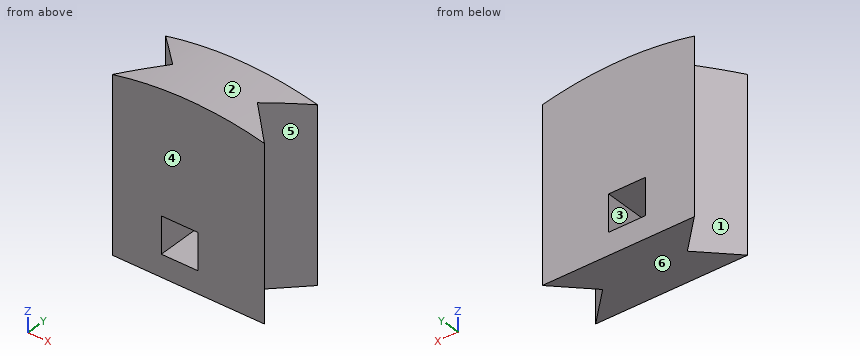
from build123d import *

# Parameters (mm, degrees)
F1_DEPTH = 47
F3_DEPTH = 25
F4_W     = 9.5
F4_H     = 9.5
F5_DEPTH = 25


with BuildPart() as f1:
    # F0 (on Top) → F1 (new body)
    with BuildSketch(Plane.XY):
        Polygon((8.75, 8.75), (0, 0), (39.5, 0), (30.75, 8.75), (39.5, 17.5), (0, 17.5), align=None)
    extrude(amount=F1_DEPTH)

    # F2 (on face) → F3 (cut)
    with BuildSketch(Plane.XZ):
        with BuildLine():
            ThreePointArc((-5.643996, 43.338941), (18.362093, 46.989286), (42.469436, 44.081821))
            Line((42.469436, 44.081821), (45.143996, 47.1))
            Line((45.143996, 47.1), (-5.643996, 47.1))
            Line((-5.643996, 47.1), (-5.643996, 43.338941))
        make_face()
    extrude(amount=-F3_DEPTH, mode=Mode.SUBTRACT)

    # F4 (on face) → F5 (cut)
    with BuildSketch(Plane.XZ):
        with Locations((17.5, 10.5)):
            Rectangle(F4_W, F4_H)
    extrude(amount=-F5_DEPTH, mode=Mode.SUBTRACT)


solid = f1.part
Geometry check sheet. Reference: the model listing, model coordinates, mm. Face numbers are marked on the shaded views. A direction names the side the tool comes from. Round coordinates to 2 decimals unless told otherwise and drop trailing zeros. Order: outer loops, then holes, each group sorted by start corner. A loop starts at its lowest first (then second) coordinate and runs counter-clockwise, first axis right, second up. Notation, with made-up numbers: M 11,-29 L 38,-29 A22 ccw 38,-19 Z; hole C 44,39 d3. An arc over 180 degrees is marked long. Write each question's results on one line, items separated by ' | '. Start each with the question number.
1. Go/stop test with flat-tipped pins: P1, Ø7.5, axis at y = 6, z = 8.5, coming from the -X side; P2, Ø1.5, axis at y = 6.5, z = 19, coming from the +X side; P3, Ø10.5, axis at y = 6, z = 11, coming from the +X side. Record where each tip stops, or that it passes through.
2. Draft check along Y on the marked faces 4, 5 and 6. Enter one of: pulls with the +Y half, pulls with the -Y half, needs draft (parallel to the pull), parting line crosses it, or undercut.
3. Cross-section at B-B on x = 20. Record the boundary of the cut face in (y, z).
4. Set-up check for the marked faces 1, 2 and 3: record each of +Z, -Z, +X, -X, +Y, -Y from which the full face is reachable in a straight line by a thin tool's end or side.
5. Cross-section at D-D on x = 37.5. Record the boundary of the cut face in (y, z), plus the area to 3 significant figures.
6. Material ranges on L1, parallel to X at y = 16.75, z = 12; L2, parallel to Z at x = 21, y = 1.25; L3, parallel to Y at x = 32, z = 11, recorded low to high. Write a range as from..to.
7. Cross-section at A-A on z = 10.5. Record the boundary of the cut face in (x, y), plus the area to 3 significant figures.
8. Cross-section at C-C on y = 11.5. Record the boundary of the cut face in (x, z).
Resolved:
1) P1: x = 2.25 | P2: x = 33.75 | P3: x = 38.75
2) face 4: pulls with the -Y half | face 5: undercut | face 6: needs draft
3) outline: M 0,0 L 17.5,0 L 17.5,5.75 L 0,5.75 Z; M 0,15.25 L 17.5,15.25 L 17.5,47 L 0,47 Z
4) face 1: +Z, -Z, -X | face 2: +Z, +Y, -Y | face 3: +Y, -Y
5) outline: M 0,0 L 2,0 L 2,45.23 L 0,45.23 Z; M 15.5,0 L 17.5,0 L 17.5,45.23 L 15.5,45.23 Z | area: 181 mm2
6) L1: 0.75..12.75, 22.25..38.75 | L2: 0..5.75, 15.25..46.99 | L3: 0..7.5, 10..17.5
7) outline: M 0,0 L 12.75,0 L 12.75,17.5 L 0,17.5 L 8.75,8.75 Z; M 22.25,0 L 39.5,0 L 30.75,8.75 L 39.5,17.5 L 22.25,17.5 Z | area: 372 mm2
8) outline: M 6,0 L 33.5,0 L 33.5,45.94 A89.9 ccw 6,45.94 Z; hole M 12.75,5.75 L 22.25,5.75 L 22.25,15.25 L 12.75,15.25 Z
